Source: CAD feature listing. Evaluate the final solid. Frame: model axes, mm. A direction names the side the tool comes from. Round coordinates to 2 decimals unless told otherwise and drop trailing zeros. Loops run counter-clockwise (first coordinate to the right, second up) from the corner with the lowest first, then second, coordinate; pieces in that order, holes last.
Item 1: Access query for faces 1 (the flat face through (49, 5.6, 0)), 2 (the flat face through (33, 4, 0)), 3 (the cylindrical face through (-39.14, 0.81, 14.1)), 4 (the flat face through (44, 4, 6)). Directions: +Z, -Z, +X, -X, +Y, -Y. A direction counts if a zero-diameter tool reaches every point of the face in a straight line with its end or side. Return the directions, or none.
Item 2: Section query B-B on x = -21. Return loops of the section in (y, z).
Item 3: Section query A-A on x = 44.5. Return loops of the section in (y, z), then the cut area to 3 significant figures.
Item 4: Pull-direction query (X, two-part tool) for faces 5 (the cylindrical face through (39.1, 0.81, -14.14)), 6 (the flat face through (49, 4, -5.5)), 7 (the cylindrical face through (-36.03, 0.81, 13.27)); classes: released by +X, released by -X, zero draft, split by the parting line, or undercut.
Item 5: Ray query, L1, parallel to X at y = 0.55, z = -12; L2, parallel to Z at x = 50, y = 4; L3, parallel to Y at x = -21.5, z = -7.25. Return the intervals inside material, ascending.
Item 6: First-contact query: P1, Ø12, axis at x = 47, z = 2.5, coming from the -Y side; P2, Ø12, axis at x = 4.5, z = 8, coming from the +Y side; P3, Ø3, axis at x = 28, z = 12, coming from the +Y side; P4, Ø1.4, axis at x = 51, y = 4.5, coming from the -Z side. Flat tips, straight axial feed; report the tip coordinate or a pass-through.
```python
from build123d import *

# Parameters (mm, degrees)
PCB_OUTLINE_W                  = 80
PCB_OUTLINE_H                  = 30
PCB_BASE_DEPTH                 = 1.6
SKETCH3_W                      = 22
SKETCH3_H                      = 12
USB_CONNECTTOR_DUMMY_DEPTH     = 4.5
HOLE_LOCATIONS_R               = 1.6
MOUNTING_HOLES_DEPTH           = 58.18609971
SKETCH4_W                      = 11
SKETCH4_H                      = 3.5
SKETCH4_W_2                    = 10
SKETCH4_H_2                    = 1.25
USB_CONNECTOR_DUMMY_HOLE_DEPTH = 12
FILLET1_R                      = 3
SKETCH5_W                      = 1.5
SKETCH5_H                      = 1.5
CUT_EXTRUDE1_DEPTH             = 0.5


with BuildPart() as part:
    # PCB_Outline → PCB_Base (new body)
    with BuildSketch(Plane(origin=(0, 0, 0), x_dir=(1, 0, 0), z_dir=(0, 1, 0))):
        Rectangle(PCB_OUTLINE_W, PCB_OUTLINE_H)
    extrude(amount=PCB_BASE_DEPTH)

    # Sketch3 → USB_Connecttor_Dummy (add)
    with BuildSketch(Plane(origin=(0, 1.6, 0), x_dir=(1, 0, 0), z_dir=(0, 1, 0))):
        with Locations((44, 0)):
            Rectangle(SKETCH3_W, SKETCH3_H)
    extrude(amount=USB_CONNECTTOR_DUMMY_DEPTH)

    # Hole_Locations → Mounting_Holes (cut, through all)
    with BuildSketch(Plane(origin=(0, 1.6, 0), x_dir=(1, 0, 0), z_dir=(0, 1, 0))):
        with Locations(Location((-37, 12, 0), (0, 0, 270))):
            Circle(HOLE_LOCATIONS_R)
        with Locations(Location((28, 12, 0), (0, 0, 270))):
            Circle(HOLE_LOCATIONS_R)
        with Locations(Location((-37, -12, 0), (0, 0, 90))):
            Circle(HOLE_LOCATIONS_R)
        with Locations(Location((28, -12, 0), (0, 0, 90))):
            Circle(HOLE_LOCATIONS_R)
    extrude(amount=-MOUNTING_HOLES_DEPTH, mode=Mode.SUBTRACT)

    # Sketch4 → USB_Connector_Dummy_Hole (cut)
    with BuildSketch(Plane(origin=(55, 0, 0), x_dir=(0, 0, -1), z_dir=(1, 0, 0))):
        with Locations((0, 3.85)):
            Rectangle(SKETCH4_W, SKETCH4_H)
        with Locations((0, 4.475)):
            Rectangle(SKETCH4_W_2, SKETCH4_H_2, mode=Mode.SUBTRACT)
    extrude(amount=-USB_CONNECTOR_DUMMY_HOLE_DEPTH, mode=Mode.SUBTRACT)

    # Fillet1
    fillet1_edges = [part.edges().sort_by_distance(p)[0] for p in [
        (40, 0.8, 15),
        (-40, 0.8, 15),
        (-40, 0.8, -15),
        (40, 0.8, -15),
    ]]
    fillet(fillet1_edges, radius=FILLET1_R)

    # Sketch5 → Cut-Extrude1 (cut)
    with BuildSketch(Plane.XZ.offset(-1.6)):
        with Locations((50.25, -2.75)):
            Rectangle(SKETCH5_W, SKETCH5_H)
        with Locations((50.25, 2.75)):
            Rectangle(SKETCH5_W, SKETCH5_H)
    extrude(amount=-CUT_EXTRUDE1_DEPTH, mode=Mode.SUBTRACT)


solid = part.part
```
Data:
1. face 1: +X
1. face 2: +Z, -Z, -X, +Y
1. face 3: +Z, -X, +Y, -Y
1. face 4: +Z, +X, -X, +Y
2. outline: (0, -15) - (1.6, -15) - (1.6, 15) - (0, 15) - close
3. outline: (1.6, -6) - (6.1, -6) - (6.1, 6) - (1.6, 6) - close; (3.85, -5) - (5.1, -5) - (5.1, 5) - (3.85, 5) - close; hole (2.1, -5.5) - (5.6, -5.5) - (5.6, 5.5) - (2.1, 5.5) - close
3. area: 28.0 mm2
4. face 5: released by +X
4. face 6: zero draft
4. face 7: undercut
5. L1: x = -40 to -38.6, -35.4 to 26.4, 29.6 to 40
5. L2: z = -6 to -5.5, -5 to 5, 5.5 to 6
5. L3: y = 0 to 1.6
6. P1: stops at y = 1.6
6. P2: stops at y = 1.6
6. P3: passes through
6. P4: stops at z = -6
